CAD build for the part. Positions are in the model's coordinates, mm. Face numbers are marked on the shaded views. A direction names the side the tool comes from. Coordinates: 2 decimals unless noted, no trailing zeros. Order: outer loops, then holes, each group sorted by start corner. A loop starts at its lowest first (then second) coordinate and runs counter-clockwise, first axis right, second up.
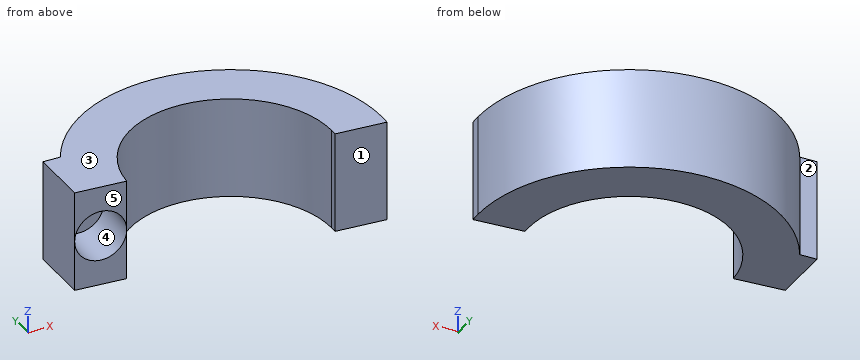
from build123d import *

# Parameters (mm, degrees)
F1_DEPTH = 12.7
F3_DEPTH = 6.35


with BuildPart() as f1:
    # F0 (on Top) → F1 (new body)
    with BuildSketch(Plane.XY):
        with BuildLine():
            Line((-19.0055783398, 41.7074999772), (-25.3555783398, 41.7074999772))
            Line((-25.3555783398, 41.7074999772), (-19.0203855599, 41.2741035754))
            ThreePointArc((-19.0203855599, 41.2741035754), (-5.9163507237, 53.0999050026), (6.35, 40.4073107719))
            ThreePointArc((6.35, 40.4073107719), (6.3425942307, 39.9736614957), (6.3203855599, 39.5405179684))
            Line((6.3203855599, 39.5405179684), (12.6555783398, 39.1071215667))
            ThreePointArc((12.6555783398, 39.1071215667), (12.688891346, 39.7568368575), (12.7, 40.4073107719))
            ThreePointArc((12.7, 40.4073107719), (-1.7541560784, 58.8946231415), (-23.1824901468, 49.3274999772))
            Line((-23.1824901468, 49.3274999772), (-19.0055783398, 49.3274999772))
            Line((-19.0055783398, 49.3274999772), (-19.0055783398, 41.7074999772))
        make_face()
        with BuildLine():
            ThreePointArc((-23.1824901468, 49.3274999772), (-24.6696039317, 45.6317353132), (-25.3555783398, 41.7074999772))
            Line((-25.3555783398, 41.7074999772), (-19.0055783398, 41.7074999772))
            Line((-19.0055783398, 41.7074999772), (-19.0055783398, 49.3274999772))
            Line((-19.0055783398, 49.3274999772), (-23.1824901468, 49.3274999772))
        make_face()
        with BuildLine():
            Line((-25.3555783398, 49.3274999772), (-25.3555783398, 41.7074999772))
            ThreePointArc((-25.3555783398, 41.7074999772), (-24.6696039317, 45.6317353132), (-23.1824901468, 49.3274999772))
            Line((-23.1824901468, 49.3274999772), (-25.3555783398, 49.3274999772))
        make_face()
    extrude(amount=F1_DEPTH)

    # F2 (on face) → F3 (cut)
    with BuildSketch(Plane(origin=(2.7218447995, 39.7866974726, 0), x_dir=(0.9976681543, -0.0682514019, 0), z_dir=(-0.0682514019, -0.9976681543, 0))):
        with BuildLine():
            ThreePointArc((-21.7930483851, 6.35), (-24.9680483851, 9.525), (-28.1430483851, 6.35))
            ThreePointArc((-28.1430483851, 6.35), (-24.9680483851, 3.175), (-21.7930483851, 6.35))
        make_face()
    extrude(amount=-F3_DEPTH, mode=Mode.SUBTRACT)


solid = f1.part
1) Drill centre lines: probe 1 along X at (y, z) = (47.5, 9); probe 2 along X at (y, z) = (49.5, 1.5); probe 3 along X at (y, z) = (50, 8.25). Where is each one in solid material? Low to high.
2) Slice it at D-D (y = 56). List the corners of the cut face in (x, z), plus the area to 3 significant figures.
3) Pin check, flat tips, straight feed: P1, Ø1.1, axis at x = -24, z = 4.5, coming from the +Y side; P2, Ø1, axis at x = -19, z = 6.5, coming from the -Y side; P3, Ø5, axis at x = -3.5, z = 2, coming from the -Y side; P4, Ø12, axis at x = -0.5, y = 43, coming from the +Z side. Stop position of each tip, or through.
4) Which spindle directions (+Z, -Z, +X, -X, +Y, -Y) get a long thin tool onto all of the face, cutting with end or side? Do the marked faces 1 and 2. Say none if no direction does.
5) Slice it at C-C (x = -6.35). List the corners of the cut face in (y, z).
6) Slice it at B-B (y = 52.25). List the corners of the cut face in (x, z).
7) Two-plate mould, pull along Z, no slides. Class the marked faces 3, 4 and 5: released by +Z, released by -Z, zero draft, split by the parting line, or undercut.
Worked out:
1. probe 1: x = -25.36 to -23.53, -20.02 to -16.88, 4.18 to 11.33
1. probe 2: x = -23.09 to -15.22, 2.52 to 10.39
1. probe 3: x = -22.81 to -14.67, 1.97 to 10.11
2. outline: (-17.29, 0) - (4.59, 0) - (4.59, 12.7) - (-17.29, 12.7) - close
2. area: 278 mm2
3. P1: stops at y = 49.33
3. P2: stops at y = 41.27
3. P3: stops at y = 51.93
3. P4: passes through
4. face 1: +Z, -Z, -X, -Y
4. face 2: +Z, -Z, -X, +Y
5. outline: (53.11, 0) - (59.46, 0) - (59.46, 12.7) - (53.11, 12.7) - close
6. outline: (-21.27, 0) - (-10.94, 0) - (-10.94, 12.7) - (-21.27, 12.7) - close; (-1.76, 0) - (8.57, 0) - (8.57, 12.7) - (-1.76, 12.7) - close
7. face 3: released by +Z
7. face 4: undercut
7. face 5: zero draft
